```python
from build123d import *

# Parameters (mm, degrees)
F0_R     = 2.5
F1_DEPTH = 10
F3_DEPTH = 5
F5_D     = 2
F5_DEPTH = 1
F5_TIP   = 0.600860619


with BuildPart() as f1:
    # F0 (on Top) → F1 (new body)
    with BuildSketch(Plane.XY):
        Circle(F0_R)
    extrude(amount=F1_DEPTH)

    # F2 (on face) → F3 (cut)
    with BuildSketch(Plane.XY.offset(10)):
        Polygon((1.5, -0.8660254038), (1.5, 0.8660254038), (0, 1.7320508076), (-1.5, 0.8660254038), (-1.5, -0.8660254038), (0, -1.7320508076), align=None)
    extrude(amount=-F3_DEPTH, mode=Mode.SUBTRACT)

    # F5
    with Locations(Plane(origin=(0, 0, 0), x_dir=(1, 0, 0), z_dir=(0, 0, -1))):
        with Locations((0, 0)):
            Hole(F5_D / 2, depth=F5_DEPTH)
            with Locations((0, 0, -(F5_DEPTH + F5_TIP / 2))):  # 118° drill point
                Cone(0, F5_D / 2, F5_TIP, mode=Mode.SUBTRACT)


solid = f1.part
```
The listing builds one solid part. Answer for the finished solid, in the listing's coordinates (mm). A direction names the side the tool comes from. Round coordinates to 2 decimals unless told otherwise and drop trailing zeros. Loops run counter-clockwise (first coordinate to the right, second up) from the corner with the lowest first, then second, coordinate; pieces in that order, holes last. Notation, with made-up numbers: (-34, 85.25) - (24, 85.25) arc R14 ccw to (24, 109.25) - close; hole circle Ø3 at (63.5, 88.25). An arc over 180 degrees is marked (long way). Use one line per item in the form item = value. Start each with the question number.
1. The part is cut by section B-B on y = 1.35. Determine the outline of the cut face in (x, z), then the cut area to 3 significant figures.
2. The part is cut by section C-C on x = 1.1. Determine the outline of the cut face in (y, z) (3 decimals), then the cut area to 3 significant figures.
3. For a pull along Y with two mould halves and no side action, classify faces 1 (the face through (1.5, 0, 8)), 2 (the face through (2, 0, 10)), 3 (the face through (-0.54, -2.44, 4.93)) as pulls with the +Y half, pulls with the -Y half, needs draft (parallel to the pull), parting line crosses it, or undercut.
4. Consider line 1 (Y direction, x = 0, z = 0.6); line 2 (Z direction, x = -1.1, y = -0.3); line 3 (X direction, y = -2, z = 6.5). Determine where each line is inside the solid, lowest interval first. Write a range as [from, to].
5. The part is cut by section A-A on z = 7.25. Determine the outline of the cut face in (x, y).
6. Given pin 1 Ø0.9 at (y, z) = (0.5, 7) entering from +X; pin 2 Ø2.5 at (x, y) = (0, 0) entering from +Z; pin 3 Ø1 at (y, z) = (-1.5, 4.5) entering from +X; pin 4 Ø1 at (x, z) = (1, 2) entering from -Y, each flat-ended and moving along its own axis, determine where each tip first touches the part or whether it passes through.
7. A tool of negligible diameter and unlimited length cuts with its end or side. For faces 4 (the face through (-1.5, 0, 8)), 5 (the face through (1, -1, 0)), 6 (the face through (0.217, 0.976, 0.507)), from which of +Z, -Z, +X, -X, +Y, -Y can it reach the whole face along a straight path? Write none if from no direction.
8. The part is cut by section D-D on z = 2.75. Determine the outline of the cut face in (x, y), then the cut area to 3 significant figures.
Geometry check:
q1.outline = (-2.1, 0) - (2.1, 0) - (2.1, 10) - (0.66, 10) - (0.66, 5) - (-0.66, 5) - (-0.66, 10) - (-2.1, 10) - close
q1.area = 35.5 mm^2
q2.outline = (-2.245, 0) - (2.245, 0) - (2.245, 10) - (1.097, 10) - (1.097, 5) - (-1.097, 5) - (-1.097, 10) - (-2.245, 10) - close
q2.area = 33.9 mm^2
q3.face_1 = undercut
q3.face_2 = needs draft
q3.face_3 = parting line crosses it
q4.line_1 = [-2.5, -1], [1, 2.5]
q4.line_2 = [0, 5]
q4.line_3 = [-1.5, 1.5]
q5.outline = circle Ø5 at (0, 0); hole (-1.5, -0.87) - (0, -1.73) - (1.5, -0.87) - (1.5, 0.87) - (0, 1.73) - (-1.5, 0.87) - close
q6.pin_1 = 2.5
q6.pin_2 = 5
q6.pin_3 = 2.29
q6.pin_4 = -2.45
q7.face_4 = +Z
q7.face_5 = -Z, +X, -X, +Y, -Y
q7.face_6 = -Z
q8.outline = circle Ø5 at (0, 0)
q8.area = 19.6 mm^2
